Source: three-view drawing plus pictorial views. Frame: mm from the lowest corner of the part. Give positions to 0.01 mm unless a question says otherwise; leave off trailing zeros. Loops run counter-clockwise (first coordinate to the right, second up) from the corner with the lowest first, then second, coordinate; pieces in that order, holes last. Notation, with made-up numbers: (12.5, 74) - (60.5, 74) arc R25 ccw to (60.5, 102) - close; hole circle Ø3 at (57, 25). An arc over 180 degrees is marked (long way). Answer in a Markdown table with one row per item.
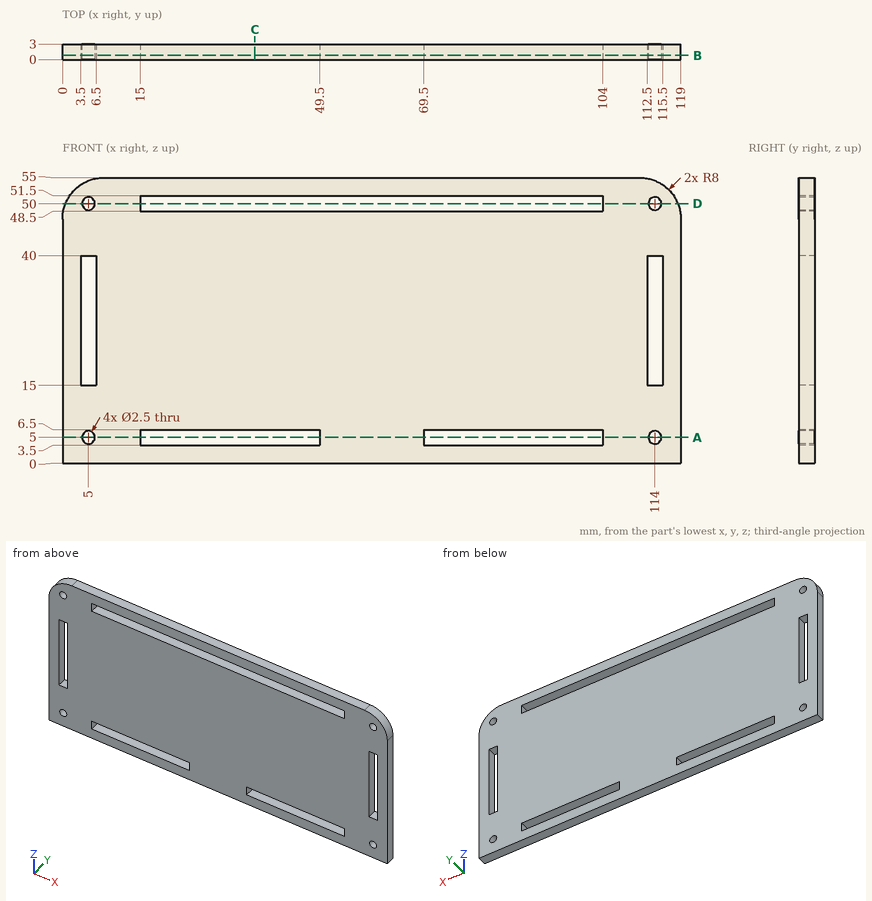
Q1. Cut plane A-A (z = 5). Output: boundary loops of the cut face in (x, y), and give its area (3 significant figures).
Check values:
| item | result |
|---|---|
| outline | (0, 0) - (3.75, 0) - (3.75, 3) - (0, 3) - close; (6.25, 0) - (15, 0) - (15, 3) - (6.25, 3) - close; (49.5, 0) - (69.5, 0) - (69.5, 3) - (49.5, 3) - close; (104, 0) - (112.75, 0) - (112.75, 3) - (104, 3) - close; (115.25, 0) - (119, 0) - (119, 3) - (115.25, 3) - close |
| area | 135 mm² |
Q2. Cut plane B-B (y = 0.8). Give the number of separate pieces and of enclosed holes in the cut face, and give its area (3 significant figures).
Check values:
| item | result |
|---|---|
| separate pieces | 1 |
| enclosed holes | 9 |
| area | 5,870 mm² |
Q3. Cut plane C-C (x = 37). Output: boundary loops of the cut face in (y, z), and give its area (3 significant figures).
Check values:
| item | result |
|---|---|
| outline | (0, 0) - (3, 0) - (3, 3.5) - (0, 3.5) - close; (0, 6.5) - (3, 6.5) - (3, 48.5) - (0, 48.5) - close; (0, 51.5) - (3, 51.5) - (3, 55) - (0, 55) - close |
| area | 147 mm² |
Q4. Cut plane D-D (z = 50). Output: boundary loops of the cut face in (x, y), and give its area (3 significant figures).
Check values:
| item | result |
|---|---|
| outline | (0.58, 0) - (3.75, 0) - (3.75, 3) - (0.58, 3) - close; (6.25, 0) - (15, 0) - (15, 3) - (6.25, 3) - close; (104, 0) - (112.75, 0) - (112.75, 3) - (104, 3) - close; (115.25, 0) - (118.42, 0) - (118.42, 3) - (115.25, 3) - close |
| area | 71.5 mm² |
Q5. First-contact query: pin 1 (1.5 mm diameter, centred on y = 1, z = 49.5, fed in from -X); pin 2 (0.9 mm diameter, centred on x = 61.5, y = 1, fed in from -Z); pin 3 (1.5 mm diameter, centred on y = 0.5, z = 49, fed in from +X); pin 4 (0.9 mm diameter, centred on x = 114, y = 1, fed in from +Z). Flat tips, straight axial feed; report the tip coordinate or a pass-through.
Check values:
| item | result |
|---|---|
| pin 1 | x = 0.19 |
| pin 2 | z = 0 |
| pin 3 | x = 118.9 |
| pin 4 | z = 54.58 |
Q6. Material intervals for line 1 along X through (y, z) = (2.6, 19); line 2 along Z through (x, y) = (103, 0.55); line 3 along Z through (x, y) = (5, 2.25), sorted ascending.
Check values:
| item | result |
|---|---|
| line 1 | 0 to 3.5, 6.5 to 112.5, 115.5 to 119 |
| line 2 | 0 to 3.5, 6.5 to 48.5, 51.5 to 55 |
| line 3 | 0 to 3.75, 6.25 to 15, 40 to 48.75, 51.25 to 54.42 |
